Autodesk Inventor part; units mm, degrees
ref_plane "YZ Plane" through (0, 0, 0) normal (1, 0, 0) x (0, 1, 0)
ref_plane "XZ Plane" through (0, 0, 0) normal (0, 1, 0) x (-1, 0, 0)
ref_plane "XY Plane" through (0, 0, 0) normal (0, 0, 1) x (1, 0, 0)
sketch "Sketch1" plane through (0, 0, 0) normal (1, 0, 0) x (0, 1, 0)
  circle A0 centre (7.0357, 7.0379) radius 4.5 construction
  circle A1 centre (222.967, 132.9623) radius 4.5 construction
  arc A2 (216.9926, 130.402) -> (220.4062, 126.988) centre (222.967, 132.9623) ccw construction
  arc A3 (226.4665, 117.7965) -> (220.4062, 126.988) centre (216.4665, 117.7968) ccw construction
  line L0 (226.4665, 117.7965) -> (226.4629, 22.2035) construction
  arc A4 (220.402, 13.0124) -> (226.4629, 22.2035) centre (216.4629, 22.2039) ccw construction
  arc A5 (220.402, 13.0124) -> (216.9879, 9.5985) centre (222.9623, 7.0379) ccw construction
  arc A6 (207.7966, 3.5379) -> (216.9879, 9.5985) centre (207.7966, 13.5379) ccw construction
  line L1 (207.7966, 3.5379) -> (22.2015, 3.5379) construction
  arc A7 (13.0101, 9.5985) -> (22.2015, 3.5379) centre (22.2015, 13.5379) ccw construction
  arc A8 (13.0101, 9.5985) -> (10.3808, 12.6111) centre (7.0357, 7.0379) ccw construction
  line L2 (10.3808, 12.6111) -> (3.8893, 12.6111) construction
  line L3 (3.8893, 12.6111) -> (0, 16.5)
  line L4 (0, 16.5) -> (0, 0)
  line L5 (0, 0) -> (230, 0)
  line L6 (230, 0) -> (230.0052, 140)
  line L7 (230.0052, 140) -> (127.855, 140.0038)
  arc A9 (122.0443, 130.7772) -> (127.855, 140.0038) centre (125.5635, 135.0039) ccw
  line L8 (122.0443, 130.7772) -> (119.5403, 128.2731)
  arc A10 (119.5403, 128.2731) -> (128.6878, 126.5292) centre (125.5635, 135.0039) ccw
  arc A11 (136.9343, 125.9261) -> (128.6878, 126.5292) centre (132.1469, 117.1465) ccw construction
  arc A12 (136.9343, 125.9261) -> (146.2191, 129.5969) centre (140.0462, 131.6328) ccw construction
  arc A13 (155.7163, 136.4648) -> (146.2191, 129.5969) centre (155.716, 126.4648) ccw construction
  line L9 (155.7163, 136.4648) -> (207.8014, 136.4629) construction
  arc A14 (216.9926, 130.402) -> (207.8014, 136.4629) centre (207.801, 126.4629) ccw construction
  circle A15 centre (222.9623, 7.0379) radius 4.5 construction
  circle A16 centre (140.0462, 131.6328) radius 4.5 construction
  arc A17 (184.962, 3.5379) -> (165.0484, 3.5379) centre (175.0052, 35) ccw construction
  line L10 (184.962, 3.5379) -> (226.4622, 3.5379) construction
  line L11 (226.4622, 3.5379) -> (226.4634, 35.0003) construction
  arc A18 (223.4634, 32.0004) -> (226.4634, 35.0003) centre (223.4634, 35.0004) ccw construction
  line L12 (223.4634, 32.0004) -> (213.4634, 32.0004) construction
  arc A19 (213.4634, 38.0004) -> (213.4634, 32.0004) centre (213.4634, 35.0004) ccw construction
  line L13 (213.4634, 38.0004) -> (223.4634, 38.0004) construction
  arc A20 (226.4634, 35.0003) -> (223.4634, 38.0004) centre (223.4634, 35.0004) ccw construction
  line L14 (226.4634, 35.0003) -> (226.4647, 70.0003) construction
  arc A21 (223.4647, 67.0004) -> (226.4647, 70.0003) centre (223.4647, 70.0004) ccw construction
  line L15 (223.4647, 67.0004) -> (213.4647, 67.0004) construction
  arc A22 (213.4647, 73.0004) -> (213.4647, 67.0004) centre (213.4647, 70.0004) ccw construction
  line L16 (213.4647, 73.0004) -> (223.4647, 73.0004) construction
  arc A23 (226.4647, 70.0003) -> (223.4647, 73.0004) centre (223.4647, 70.0004) ccw construction
  line L17 (226.4647, 70.0003) -> (226.466, 105.0003) construction
  arc A24 (223.466, 102.0004) -> (226.466, 105.0003) centre (223.466, 105.0004) ccw construction
  line L18 (223.466, 102.0004) -> (213.466, 102.0004) construction
  arc A25 (213.466, 108.0004) -> (213.466, 102.0004) centre (213.466, 105.0004) ccw construction
  line L19 (213.466, 108.0004) -> (223.466, 108.0004) construction
  arc A26 (226.466, 105.0003) -> (223.466, 108.0004) centre (223.466, 105.0004) ccw construction
  line L20 (226.466, 105.0003) -> (226.4672, 136.4622) construction
  line L21 (226.4672, 136.4622) -> (145.4199, 136.4652) construction
  arc A27 (145.4199, 136.4652) -> (133.0261, 129.9155) centre (145.4194, 121.4652) ccw construction
  arc A28 (119.5403, 128.2731) -> (133.0261, 129.9155) centre (125.5635, 135.0039) ccw construction
  line L22 (119.5403, 128.2731) -> (3.8893, 12.6111)
  line L23 (3.8893, 12.6111) -> (3.5357, 12.9646)
  line L24 (3.5357, 12.9646) -> (3.5357, 3.5379) construction
  line L25 (3.5357, 3.5379) -> (165.0484, 3.5379) construction
  circle A29 centre (7.0357, 7.0379) radius 2.75
  circle A30 centre (222.9623, 7.0379) radius 2.75
  circle A31 centre (222.967, 132.9623) radius 2.75
  circle A32 centre (140.0462, 131.6328) radius 2.75
  dimension "d0" = 5.5
  dimension "d1" = 5.5
  dimension "d2" = 5.5
  dimension "d3" = 5.5
extrude "Extrusion1" add sketch "Sketch1" along normal blind 4
sketch "Sketch2" plane through (4, 0, 0) normal (1, 0, 0) x (0, 0, -1)
  line L0 (0, 0) -> (0, 230)
  line L1 (0, 230) -> (-140, 230.0052)
  line L2 (-140, 230.0052) -> (-140.0038, 127.855)
  arc A0 (-130.7772, 122.0443) -> (-140.0038, 127.855) centre (-135.0039, 125.5635) ccw
  line L3 (-130.7772, 122.0443) -> (-12.6111, 3.8893)
  line L4 (-12.6111, 3.8893) -> (-16.5, 0)
  line L5 (-16.5, 0) -> (0, 0)
  circle A1 centre (-7.0379, 7.0357) radius 2.75
  circle A2 centre (-7.0379, 222.9623) radius 2.75
  circle A3 centre (-132.9623, 222.967) radius 2.75
  circle A4 centre (-131.6328, 140.0462) radius 2.75
  circle A5 centre (-131.6328, 140.0462) radius 2.75
  circle A6 centre (-131.6328, 140.0462) radius 4.5
  circle A7 centre (-132.9623, 222.967) radius 2.75
  circle A8 centre (-132.9623, 222.967) radius 4.5
  circle A9 centre (-7.0379, 222.9623) radius 4.5
  circle A10 centre (-7.0379, 7.0357) radius 2.75
  circle A11 centre (-7.0379, 7.0357) radius 4.5
  dimension "d6" = 9
  dimension "d7" = 9
  dimension "d8" = 9
  dimension "d9" = 9
extrude "Extrusion2" add sketch "Sketch2" along normal blind 4 contours L5 L4 L3 A0 L2 L1 L0
sketch "Sketch3" plane through (8, 0, 0) normal (1, 0, 0) x (0, 0, -1)
  line L0 (0, 0) -> (0, 230) construction
  line L1 (0, 60) -> (-140.0064, 60.0052) construction
  line L2 (-140, 230.0052) -> (-140.0038, 127.855) construction
  line L3 (-127.855, 140.0038) -> (-230.0052, 140) construction
  line L4 (-210.0052, 140.0007) -> (-210.0052, 0) construction
  line L5 (-230, 0) -> (0, 0) construction
  circle A0 centre (-35, 60.0013) radius 13.5
  line L6 (-57.0351, 47.3513) -> (-57.0351, 72.6513)
  line L7 (-57.0351, 72.6513) -> (-14.4833, 72.6513)
  line L8 (-14.4833, 72.6513) -> (-14.4833, 47.3513)
  line L9 (-14.4833, 47.3513) -> (-57.0351, 47.3513)
  line L10 (-3.55, 0) -> (-3.55, 230) construction
  point P0 (-187.6552, 39.7146)
  point P1 (-187.6552, 30.2854)
  point P2 (-162.3552, 30.2854)
  point P3 (-162.3552, 39.7146)
  point P4 (-39.7146, 47.3513)
  point P5 (-30.2854, 47.3513)
  point P6 (-30.2854, 72.6513)
  point P7 (-39.7146, 72.6513)
  dimension "d12" = 60
  dimension "d13" = 20
  dimension "d14" = 27
  dimension "d17" = 25.3
  dimension "d18" = 0.85
  dimension "d19" = 3.55
  dimension "d20" = 22.0352
  dimension "d21" = 42.5518
  dimension "d22" = 21.5
extrude "Extrusion3" cut sketch "Sketch3" against normal up to next contours A0 L9 L7
sketch "Sketch4" plane through (0, 0, 0) normal (-1, 0, 0) x (0, 0, 1)
  line L0 (30.2854, 72.6513) -> (39.7146, 72.6513) construction
  line L1 (35, 72.6513) -> (35, 47.3513) construction
  line L2 (30.2854, 47.3513) -> (39.7146, 47.3513) construction
  circle A0 centre (35, 60.0013) radius 18.5
  point P0 (0, 0)
  dimension "d25" = 37
extrude "Extrusion4" cut sketch "Sketch4" against normal blind 4
fillet "Fillet1" radius 4 1 edges at (0, 60.0013, 16.5)
equation "\"d1\" = d0"
equation "\"d2\" = d0"
equation "\"d3\" = d0"
equation "\"d7\" = d6"
equation "\"d8\" = d6"
equation "\"d9\" = d6"
equation "\"d18\" = -0.5 * d17 + 0.5 * d14"
properties part number "Operator Junction Box Side Panel"
Design review of the part built by this model. Coordinates are the model's own, in mm. A direction names the side the tool comes from. Give positions to 0.01 mm unless a question says otherwise; leave off trailing zeros. Return JSON: item names as keys, results as strings. Group by question number.
Item 1: Mouldability with a two-part tool opening along Z and no side actions: class faces 1 (the flat face through (4, 113, 0)), 2 (the flat face through (4, 0, 8)), 3 (the cylindrical face through (5.972, 227.355, 8.013)) as released by +Z, released by -Z, zero draft, split by the parting line, or undercut.
Item 2: Insertion check: pin 1 Ø4.5 at (x, z) = (5.5, 35) entering from -Y; pin 2 Ø1.5 at (x, y) = (1, 103.5) entering from +Z; pin 3 Ø2.5 at (y, z) = (7, 7.5) entering from +X; pin 4 Ø1 at (x, y) = (6.5, 193) entering from +Z. Each pin has a flat end and moves straight along its axis. Give the tip position at first contact, or say it passes through.
Item 3: We need section B-B (x = 1.5). Give the number of separate pieces and of enclosed holes in the cut face, and give its area (3 significant figures).
Item 4: Tool access review of faces 4 (the flat face through (4, 46, 36)), 5 (the cylindrical face through (6, 59.8, 21.5)), 6 (the flat face through (4, 223, 4)): name each direction out of +Z, -Z, +X, -X, +Y, -Y from which nothing blocks a thin tool from reaching the whole face with its end or side.
Item 5: For probe 1 along Y at (x, z) = (2, 9); probe 2 along Z at (x, y) = (4.25, 211); probe 3 along Y at (x, z) = (2.25, 35), list the stretches that pass through material, from the lowest coordinate up.
Output:
{
 "1": {"face 1": "released by -Z", "face 2": "zero draft", "face 3": "undercut"},
 "2": {"pin 1": "stops at y = 24.03", "pin 2": "stops at z = 112.98", "pin 3": "passes through", "pin 4": "stops at z = 140"},
 "3": {"separate pieces": "1", "enclosed holes": "5", "area": "22,300 mm^2"},
 "4": {"face 4": "-X", "face 5": "+X, -X", "face 6": "+X"},
 "5": {"probe 1": "y = 0 to 5.11, 8.96 to 221.04, 224.89 to 230", "probe 2": "z = 0 to 140", "probe 3": "y = 26.28 to 41.1, 78.9 to 230"}
}
